Could you check a few things on this model? Use its own coordinates, in mm. Face numbers are marked on the shaded views. A direction names the side the tool comes from. Round coordinates to 2 decimals unless told otherwise and drop trailing zeros. Write each loop counter-clockwise with the first axis right and the second up, starting at its lowest first coordinate (ties: lowest second). Pieces come first, ordered by that corner, then holes. Notation, with made-up numbers: (53.5, 41) -> (109.5, 41) arc R14 ccw to (109.5, 50) -> close; hole circle Ø6 at (52, 14.5). An arc over 180 degrees is marked (long way). One line per question, with ' | ' between items. Start each with the question number.
1. Imagine slicing it at B-B, the plane x = 33. List the corners of the cut face in (y, z) for me, and give its area (3 significant figures).
2. For the marked faces 5 and 6, which set-ups out of +Z, -Z, +X, -X, +Y, -Y let a thin tool reach every point of the face, with its end or its side?
3. Imagine slicing it at D-D, the plane x = 52.5. State how many separate pieces and enclosed holes the cut face has, and give its area (3 significant figures).
4. Imagine slicing it at A-A, the plane y = 53.5. List the corners of the cut face in (x, z) for me, and give its area (4 significant figures).
5. Thinking about a two-plate mould opening in X: for the marked faces 1, 2, 3 and 4, which applies, released by +X, released by -X, zero draft, split by the parting line, or undercut?
6. If I drill on line 1 along Y through (x, z) = (3.5, 13.25); line 2 along X through (y, z) = (30.5, 3.75); line 3 along X through (y, z) = (4.5, 8.25), over which ranges is the centre line in solid material (lowest first)? Write a range as [from, to].
7. Imagine slicing it at C-C, the plane y = 11.5. List the corners of the cut face in (x, z) for me.
8. For pin 1 Ø2 at (x, y) = (9, 49.5) entering from -Z; pin 2 Ø2 at (x, y) = (18.5, 10) entering from +Z; pin 3 Ø1.2 at (x, y) = (20, 82.5) entering from +Z, each with a flat end and sliding along its axis, tell me the tip position at first contact or that it passes through.
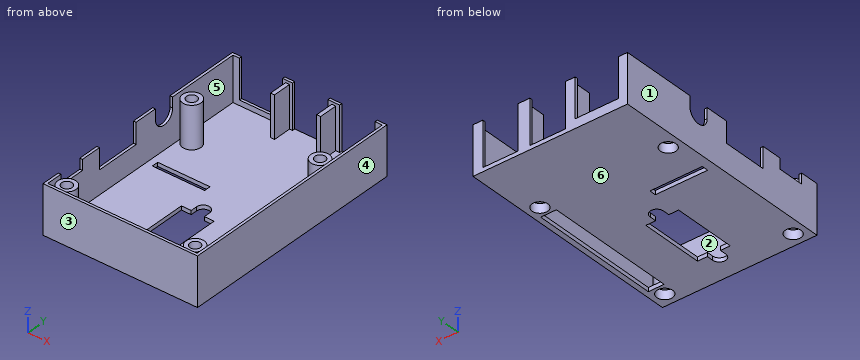
from build123d import *

# Parameters (mm, degrees)
SKETCH_W        = 59
SKETCH_H        = 88
SKETCH_R        = 2
SKETCH_W_2      = 20
SKETCH_H_2      = 2.5
SKETCH_W_3      = 6
SKETCH_H_3      = 50
PAD_DEPTH       = 18.5
SKETCH001_W     = 57
SKETCH001_H     = 86
POCKET_DEPTH    = 17
SKETCH003_W     = 16.5
SKETCH003_H     = 15
SKETCH003_W_2   = 13.5
SKETCH003_H_2   = 17
POCKET001_DEPTH = 1
SKETCH004_R     = 3.5
SKETCH004_R_2   = 2
SKETCH004_W     = 1.5
SKETCH004_H     = 7
PAD001_DEPTH    = 16
SKETCH005_W     = 10
SKETCH005_H     = 4
SKETCH005_W_2   = 17
SKETCH005_H_2   = 8
POCKET002_DEPTH = 1
SKETCH006_R     = 3
POCKET003_DEPTH = 3.5


with BuildPart() as part:
    # Sketch → Pad (new body)
    with BuildSketch(Plane.XY):
        with Locations((28, 42.5)):
            Rectangle(SKETCH_W, SKETCH_H)
        with Locations((3.5, 61.5)):
            Circle(SKETCH_R, mode=Mode.SUBTRACT)
        with Locations((52.5, 61.5)):
            Circle(SKETCH_R, mode=Mode.SUBTRACT)
        with Locations((52.5, 3.5)):
            Circle(SKETCH_R, mode=Mode.SUBTRACT)
        with Locations((3.5, 3.5)):
            Circle(SKETCH_R, mode=Mode.SUBTRACT)
        with Locations((12, 46.25)):
            Rectangle(SKETCH_W_2, SKETCH_H_2, mode=Mode.SUBTRACT)
        with BuildLine():
            Line((21.75, 34.5), (25.5, 34.5))
            Line((25.5, 37), (25.5, 34.5))
            ThreePointArc((30.5, 37), (28, 39.5), (25.5, 37))
            Line((30.5, 37), (30.5, 34.5))
            Line((30.5, 34.5), (34.25, 34.5))
            Line((34.25, 34.5), (34.25, 10.5))
            Line((34.25, 10.5), (30.5, 10.5))
            Line((30.5, 8), (30.5, 10.5))
            ThreePointArc((25.5, 8), (28, 5.5), (30.5, 8))
            Line((25.5, 8), (25.5, 10.5))
            Line((25.5, 10.5), (21.75, 10.5))
            Line((21.75, 10.5), (21.75, 34.5))
        make_face(mode=Mode.SUBTRACT)
        with Locations((52.5, 32.5)):
            Rectangle(SKETCH_W_3, SKETCH_H_3, mode=Mode.SUBTRACT)
    extrude(amount=PAD_DEPTH)

    # Sketch001 → Pocket (cut)
    with BuildSketch(Plane.XY.offset(18.5)):
        with Locations((28, 42.5)):
            Rectangle(SKETCH001_W, SKETCH001_H)
    extrude(amount=-POCKET_DEPTH, mode=Mode.SUBTRACT)

    # Sketch003 → Pocket001 (cut)
    with BuildSketch(Plane(origin=(0, 86.5, 0), x_dir=(-1, 0, 0), z_dir=(0, 1, 0))):
        with Locations((-10.25, 11)):
            Rectangle(SKETCH003_W, SKETCH003_H)
        with Locations((-29, 10)):
            Rectangle(SKETCH003_W_2, SKETCH003_H_2)
        with Locations((-47, 10)):
            Rectangle(SKETCH003_W_2, SKETCH003_H_2)
    extrude(amount=-POCKET001_DEPTH, mode=Mode.SUBTRACT)

    # Sketch004 → Pad001 (new body)
    with BuildSketch(Plane.XY.offset(1.5)):
        with Locations((3.5, 61.5)):
            Circle(SKETCH004_R)
        with Locations((3.5, 61.5)):
            Circle(SKETCH004_R_2, mode=Mode.SUBTRACT)
        with Locations((52.5, 61.5)):
            Circle(SKETCH004_R)
        with Locations((52.5, 61.5)):
            Circle(SKETCH004_R_2, mode=Mode.SUBTRACT)
        with Locations((52.5, 3.5)):
            Circle(SKETCH004_R)
        with Locations((52.5, 3.5)):
            Circle(SKETCH004_R_2, mode=Mode.SUBTRACT)
        with Locations((3.5, 3.5)):
            Circle(SKETCH004_R)
        with Locations((3.5, 3.5)):
            Circle(SKETCH004_R_2, mode=Mode.SUBTRACT)
        with Locations((20.375, 82)):
            Rectangle(SKETCH004_W, SKETCH004_H)
        with Locations((38, 82)):
            Rectangle(SKETCH004_W, SKETCH004_H)
    extrude(amount=PAD001_DEPTH)

    # Sketch005 → Pocket002 (cut)
    with BuildSketch(Plane(origin=(-1.5, 0, 0), x_dir=(0, -1, 0), z_dir=(-1, 0, 0))):
        with Locations((-10.6, 16.5)):
            Rectangle(SKETCH005_W, SKETCH005_H)
        with Locations((-32, 14.5)):
            Rectangle(SKETCH005_W_2, SKETCH005_H_2)
        with BuildLine():
            Line((-57.5, 18.5), (-49.5, 18.5))
            Line((-49.5, 18.5), (-49.5, 14.5))
            ThreePointArc((-57.5, 14.5), (-53.5, 10.5), (-49.5, 14.5))
            Line((-57.5, 14.5), (-57.5, 18.5))
        make_face()
    extrude(amount=-POCKET002_DEPTH, mode=Mode.SUBTRACT)

    # Sketch006 → Pocket003 (cut)
    with BuildSketch(Plane(origin=(0, 0, 0), x_dir=(1, 0, 0), z_dir=(0, 0, -1))):
        with Locations((3.5, -3.5)):
            Circle(SKETCH006_R)
        with Locations((52.5, -3.5)):
            Circle(SKETCH006_R)
        with Locations((52.5, -61.5)):
            Circle(SKETCH006_R)
        with Locations((3.5, -61.5)):
            Circle(SKETCH006_R)
    extrude(amount=-POCKET003_DEPTH, mode=Mode.SUBTRACT)


solid = part.part
Geometry results:
1) outline: (-1.5, 0) -> (10.5, 0) -> (10.5, 1.5) -> (-0.5, 1.5) -> (-0.5, 18.5) -> (-1.5, 18.5) -> close; (34.5, 0) -> (86.5, 0) -> (86.5, 1.5) -> (34.5, 1.5) -> close | area: 113 mm2
2) face 5: +Z | face 6: -Z, +X, -X, +Y, -Y
3) separate pieces: 4 | enclosed holes: 0 | area: 144 mm2
4) outline: (-1.5, 0) -> (49.5, 0) -> (49.5, 1.5) -> (-0.5, 1.5) -> (-0.5, 10.5) -> (-1.5, 10.5) -> close; (55.5, 0) -> (57.5, 0) -> (57.5, 18.5) -> (56.5, 18.5) -> (56.5, 1.5) -> (55.5, 1.5) -> close | area: 105.5 mm2
5) face 1: released by -X | face 2: undercut | face 3: zero draft | face 4: released by +X
6) line 1: y = [-1.5, -0.5], [0, 1.5], [5.5, 7], [58, 59.5], [63.5, 65] | line 2: x = [-1.5, -0.5], [56.5, 57.5] | line 3: x = [-1.5, -0.5], [0.15, 1.77], [5.23, 6.85], [49.15, 50.77], [54.23, 55.85], [56.5, 57.5]
7) outline: (-1.5, 0) -> (21.75, 0) -> (21.75, 1.5) -> (-0.5, 1.5) -> (-0.5, 14.5) -> (-1.5, 14.5) -> close; (34.25, 0) -> (49.5, 0) -> (49.5, 1.5) -> (34.25, 1.5) -> close; (55.5, 0) -> (57.5, 0) -> (57.5, 18.5) -> (56.5, 18.5) -> (56.5, 1.5) -> (55.5, 1.5) -> close
8) pin 1: stops at z = 0 | pin 2: stops at z = 1.5 | pin 3: stops at z = 17.5
